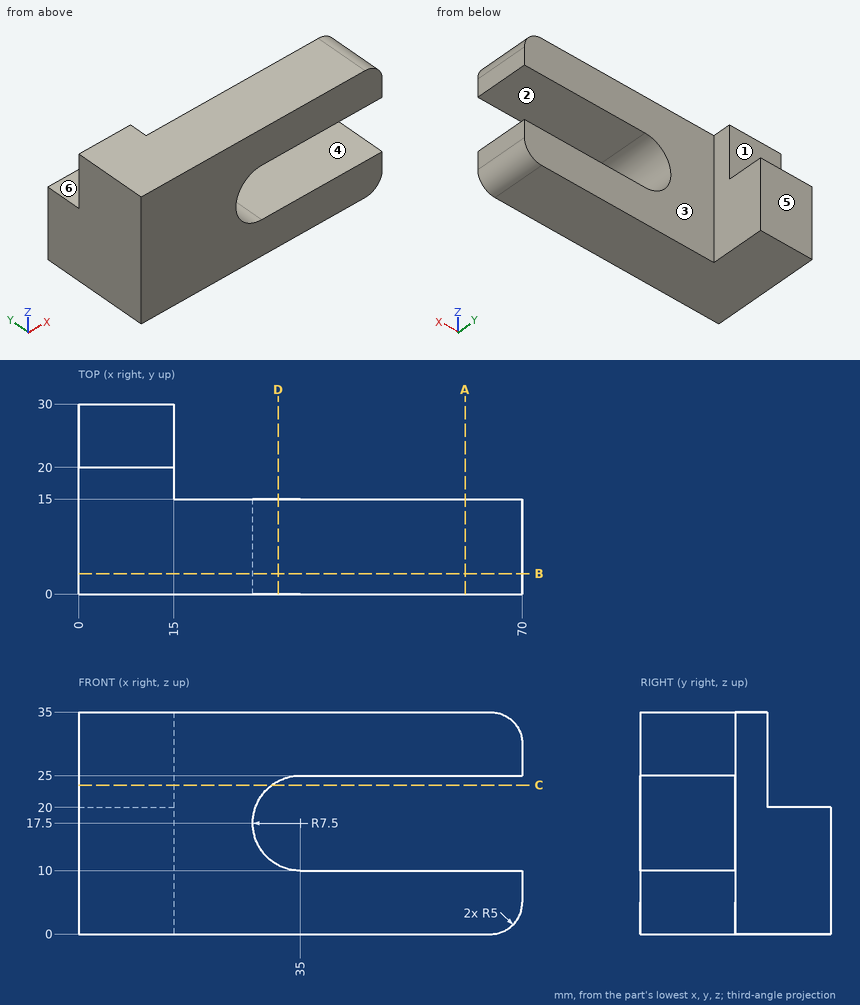
Source: three-view drawing plus pictorial views. Frame: mm from the lowest corner of the part. A direction names the side the tool comes from. Coordinates: 2 decimals unless noted, no trailing zeros. Write each loop counter-clockwise with the first axis right and the second up, starting at its lowest first coordinate (ties: lowest second). Pieces come first, ordered by that corner, then holes. Notation, with made-up numbers: (10.5, 54) -> (61.5, 54) arc R21 cw to (61.5, 87) -> close; hole circle Ø2 at (73, 16.25). An arc over 180 degrees is marked (long way). Write each question's results on one line, items separated by ' | '.
Item 1: Pin query (flat end, axial travel): pin 1 Ø10.5 at (x, z) = (37.5, 20) entering from +Y; pin 2 Ø4 at (y, z) = (19.5, 24) entering from +X. Return the tip coordinate at first contact, or that it passes through.
Conclusion:
pin 1: stops at y = 15 | pin 2: stops at x = 15
Item 2: Section query A-A on x = 61. Return loops of the section in (y, z).
Conclusion:
outline: (0, 0) -> (15, 0) -> (15, 10) -> (0, 10) -> close; (0, 25) -> (15, 25) -> (15, 35) -> (0, 35) -> close
Item 3: Material intervals for probe 1 along X at (y, z) = (28.75, 17); probe 2 along Z at (x, y) = (13.5, 20.75), sorted ascending.
Conclusion:
probe 1: x = 0 to 15 | probe 2: z = 0 to 20
Item 4: Section query C-C on z = 23.5. Return loops of the section in (x, y).
Conclusion:
outline: (0, 0) -> (30.5, 0) -> (30.5, 15) -> (15, 15) -> (15, 20) -> (0, 20) -> close
Item 5: Mould query, pull axis Z, two halves, no side actions, for the marked faces 4, 5 and 6. Classes: +Z half, -Z half, draft (parallel to the pull), parting line (faces both ways), or undercut.
Conclusion:
face 4: undercut | face 5: draft | face 6: +Z half
Item 6: Section query B-B on y = 3.25. Return loops of the section in (x, z).
Conclusion:
outline: (0, 0) -> (65, 0) arc R5 ccw to (70, 5) -> (70, 10) -> (35, 10) arc R7.5 cw to (35, 25) -> (70, 25) -> (70, 30) arc R5 ccw to (65, 35) -> (0, 35) -> close
Item 7: Set-up query: the marked faces 1, 2 and 3. Return all of +Z, -Z, +X, -X, +Y, -Y with unobstructed straight access to the full face (end or side cutting, diameter ignored); none if empty.
Conclusion:
face 1: +Z, +X, -X, +Y | face 2: +X, +Y, -Y | face 3: +Z, -Z, +X, +Y
Item 8: Section query D-D on x = 31.5. Return loops of the section in (y, z), plus the area to 3 significant figures.
Conclusion:
outline: (0, 0) -> (15, 0) -> (15, 10.87) -> (0, 10.87) -> close; (0, 24.13) -> (15, 24.13) -> (15, 35) -> (0, 35) -> close | area: 326 mm^2
